from build123d import *

# Parameters (mm, degrees)
F2_DEPTH = 10
F3_DEPTH = 10


with BuildPart() as f2:
    # F0 (on Front) → F2 (new body)
    with BuildSketch(Plane.XZ):
        Polygon((0, 30.096302), (0, 0), (200, 0), (200, 30.88115), (186.43856, 30.88115), (186.43856, 60.549472), (200, 60.549472), (200, 91.236152), (0, 91.236152), (0, 60.549472), (12.01473, 60.549472), (12.01473, 30.096302), align=None)
    extrude(amount=F2_DEPTH)

    # F1 (on Right) → F3 (join)
    with BuildSketch(Plane.YZ):
        Polygon((0, 30.661654), (0, 0), (200, 0), (200, 31.010987), (212.028906, 31.010987), (212.028906, 61.265942), (200, 61.265942), (200, 91.832541), (0, 91.832541), (0, 60.456097), (-12.524211, 60.456097), (-12.524211, 30.661654), align=None)
    extrude(amount=F3_DEPTH)


solid = f2.part
Geometry: final body of the model. Coordinates: model frame, mm. A direction names the side the tool comes from. Give positions to 0.01 mm unless a question says otherwise; leave off trailing zeros. Loops run counter-clockwise (first coordinate to the right, second up) from the corner with the lowest first, then second, coordinate; pieces in that order, holes last. Notation, with made-up numbers: (-9.75, 10) -> (40.25, 10) arc R19 cw to (40.25, 22) -> close; hole circle Ø10 at (62.5, 84.25). An arc over 180 degrees is marked (long way). Put each result on its own line as item: value.
1. Pin query (flat end, axial travel): P1, Ø11, axis at x = 195, y = -6.5, coming from the +Z side; P2, Ø4, axis at x = 77.5, z = 66, coming from the +Y side; P3, Ø3, axis at x = 3, y = 208, coming from the +Z side. Return the tip coordinate at first contact, or that it passes through.
Taken from the geometry:
P1: stops at z = 91.24
P2: stops at y = 0
P3: stops at z = 61.27
2. Ray query, line 1 along X through (y, z) = (187, 4); line 2 along Y through (x, z) = (55, 84). Return the intervals inside material, ascending. Write a range as [from, to].
Taken from the geometry:
line 1: x = [0, 10]
line 2: y = [-10, 0]
3. Cut plane A-A (z = 56.5). Return the cut outline in (x, y).
Taken from the geometry:
outline: (0, -12.52) -> (10, -12.52) -> (10, 212.03) -> (0, 212.03) -> close; (12.01, -10) -> (186.44, -10) -> (186.44, 0) -> (12.01, 0) -> close
4. Cut plane C-C (y = 146.5). Return the cut outline in (x, z).
Taken from the geometry:
outline: (0, 0) -> (10, 0) -> (10, 91.83) -> (0, 91.83) -> close
5. Pull-direction query (X, two-part tool) for faces 1 (the flat face through (200, -5, 76)), 2 (the flat face through (5, -6, 30.662)), 3 (the flat face through (12.015, -5, 46)); classes: released by +X, released by -X, zero draft, split by the parting line, or undercut.
Taken from the geometry:
face 1: released by +X
face 2: zero draft
face 3: undercut
6. Cut plane B-B (z = 81). Return the cut outline in (x, y).
Taken from the geometry:
outline: (0, -10) -> (200, -10) -> (200, 0) -> (10, 0) -> (10, 200) -> (0, 200) -> close
7. Set-up query: faces 4 (the flat face through (193, -5, 60.549)), 5 (the flat face through (6, -5, 30.096)), 6 (the flat face through (5, 200, 76)). Return all of +Z, -Z, +X, -X, +Y, -Y with unobstructed straight access to the full face (end or side cutting, diameter ignored); none if empty.
Taken from the geometry:
face 4: +X, +Y, -Y
face 5: -X, -Y
face 6: +Z, +X, -X, +Y
8. Cut plane D-D (x = 168). Return the cut outline in (y, z), plus the area to 3 significant figures.
Taken from the geometry:
outline: (-10, 0) -> (0, 0) -> (0, 91.24) -> (-10, 91.24) -> close
area: 912 mm2
